Autodesk Inventor part; units mm, degrees
ref_plane "XZ Plane" through (0, 0, 0) normal (0, 1, 0) x (-1, 0, 0)
ref_plane "XY Plane" through (0, 0, 0) normal (0, 0, 1) x (1, 0, 0)
sketch "Sketch1" plane through (0, 0, 0) normal (0, 1, 0) x (-1, 0, 0)
  line L0 (0, 0) -> (-330, 0)
  line L1 (-330, 0) -> (-330, 25)
  line L2 (-330, 25) -> (0, 25)
  line L3 (0, 25) -> (0, 0)
  dimension "d0" = 330
  dimension "d1" = 25
extrude "Extrusion1" add sketch "Sketch1" along normal blind 1
sketch "Sketch2" plane through (0, 1, 0) normal (0, 1, 0) x (1, 0, 0)
  line L0 (0, 0) -> (330, 0)
  line L1 (330, 0) -> (330, -1)
  line L2 (330, -1) -> (0, -1)
  line L3 (0, -1) -> (0, 0)
  dimension "d4" = 330
  dimension "d5" = 1
extrude "Extrusion2" add sketch "Sketch2" along normal blind 24
hole "Hole1" at (20, 12.4367, 1) direction (0, 0, -1) diameter 5.5 end through all
pattern_linear "Rectangular Pattern1" count 2 spacing 50 along (1, 0, 0) of "Hole1"
ref_plane "Work Plane1" through (165, 0, 0) normal (1, 0, 0) x (0, 1, 0)
mirror "Mirror1" about plane through (165, 0, 0) normal (1, 0, 0) of "Hole1", "Rectangular Pattern1"
ref_plane "Work Plane2" through (82.5, 1, 1) normal (0, -0.7071, 0.7071) x (-1, 0, 0)
mirror "Mirror2" about plane through (82.5, 1, 1) normal (0, -0.7071, 0.7071) of "Extrusion2", "Hole1", "Rectangular Pattern1", "Mirror1"
properties part number "Lbarx1 big" material "Aluminum 6061"
Model file for the job. Use its own axes, mm. A direction names the side the tool comes from. Give positions to 0.01 mm unless a question says otherwise; leave off trailing zeros. Loops run counter-clockwise (first coordinate to the right, second up) from the corner with the lowest first, then second, coordinate; pieces in that order, holes last.
1) Saw through at D-D (x = 252.5). Write the cut outline in (y, z), plus the area to 3 significant figures.
2) Wall check: line 1 (Y direction, x = 70, z = 0.65); line 2 (Y direction, x = 277.5, z = 18.75). Give the ranges that are in metal, low to high.
3) Saw through at B-B (y = 5). Write the cut outline in (x, z).
4) Saw through at A-A (x = 20). Write the cut outline in (y, z), plus the area to 3 significant figures.
5) Pull direction Z, two halves, no side cores. Call faces 1 (the flat face through (163, 12, 0)), 2 (the cylindrical face through (262.685, 13.033, 0.493)), 3 (the cylindrical face through (22.727, 0.493, 12.795)): +Z half, -Z half, draft (parallel to the pull), parting line (faces both ways), or undercut.
6) Tool access for faces 4 (the cylindrical face through (257.315, 0.493, 13.033)), 5 (the flat face through (167, 1, 13)): list every direction of +Z, -Z, +X, -X, +Y, -Y with a clear straight run to the whole face (end or side of a thin tool).
7) Flat gauge pins, fed straight in: pin 1 Ø3 at (x, y) = (87, 16.5) entering from +Z; pin 2 Ø5 at (x, y) = (260, 12.44) entering from +Z; pin 3 Ø5 at (x, z) = (92, 9.5) entering from +Y. Where does each tip first touch, or does it go through?
Answer block:
1. outline: (0, 0) - (25, 0) - (25, 1) - (1, 1) - (1, 25) - (0, 25) - close
1. area: 49.0 mm2
2. line 1: y = 0 to 9.69, 15.19 to 25
2. line 2: y = 0 to 1
3. outline: (0, 0) - (330, 0) - (330, 1) - (0, 1) - close
4. outline: (0, 0) - (9.69, 0) - (9.69, 1) - (1, 1) - (1, 9.69) - (0, 9.69) - close; (0, 15.19) - (1, 15.19) - (1, 25) - (0, 25) - close; (15.19, 0) - (25, 0) - (25, 1) - (15.19, 1) - close
4. area: 38.0 mm2
5. face 1: -Z half
5. face 2: draft
5. face 3: undercut
6. face 4: +Y, -Y
6. face 5: +Z, +X, -X, +Y
7. pin 1: stops at z = 1
7. pin 2: passes through
7. pin 3: stops at y = 1
